Design review of the part built by this model. Coordinates are the model's own, in mm. A direction names the side the tool comes from. Round coordinates to 2 decimals unless told otherwise and drop trailing zeros. Write each loop counter-clockwise with the first axis right and the second up, starting at its lowest first coordinate (ties: lowest second). Pieces come first, ordered by that corner, then holes. Notation, with made-up numbers: (78.25, 71.5) -> (83.25, 71.5) arc R18 ccw to (83.25, 99.5) -> close; hole circle Ø8 at (74, 39). An arc over 180 degrees is marked (long way). One line per question, with ' | ' between items. Start each with the question number.
1) For faces 1 (the flat face through (103, 101.6, 25)), 2 (the conical face through (17.542, 17.713, 1.708)), list the 3-axis set-ups (+Z, -Z, +X, -X, +Y, -Y) from which the entire face can be reached by the end or side of a thin tool; tool diameter is ignored.
2) Consider section B-B (x = 86.5). Give the boundary of the cut face in (y, z) (3 decimals), then the cut area to 3 significant figures.
3) For probe 1 along Z at (x, y) = (105, 25.5); probe 2 along Z at (x, y) = (78, 87.5); probe 3 along Y at (x, z) = (35, 48.5), list the stretches that pass through material, from the lowest coordinate up.
4) Insertion check: pin 1 Ø1 at (x, y) = (156, 29) entering from -Z. The pin has a flat end and moves straight along its axis. Give the tip position at first contact, or say it passes through.
5) Consider section A-A (y = 58). Give the boundary of the cut face in (x, z) (3 decimals).
6) Mouldability with a two-part tool opening along X and no side actions: class faces 3 (the flat face through (0, 51, 25)), 4 (the flat face through (100, 51, 2.032)), 5 (the flat face through (100, 51, 50.8)) as +X half, -X half, draft (parallel to the pull), parting line (faces both ways), or undercut.
```python
from build123d import *

# Parameters (mm, degrees)
F1_DEPTH = 50.8
F2_R     = 3.175
F3_R     = 3.175
F4_DEPTH = 2.032
F4_TAPER = 45


with BuildPart() as f1:
    # F0 (on Top) → F1 (new body)
    with BuildSketch(Plane.XY):
        with BuildLine():
            ThreePointArc((0, 3.175), (0.9299359697, 0.9299359697), (3.175, 0))
            Line((3.175, 0), (200.025, 0))
            ThreePointArc((200.025, 0), (202.2700640303, 0.9299359697), (203.2, 3.175))
            Line((203.2, 3.175), (203.2, 98.425))
            ThreePointArc((203.2, 98.425), (202.2700640303, 100.6700640303), (200.025, 101.6))
            Line((200.025, 101.6), (3.175, 101.6))
            ThreePointArc((3.175, 101.6), (0.9299359697, 100.6700640303), (0, 98.425))
            Line((0, 98.425), (0, 3.175))
        make_face()
        with BuildLine():
            ThreePointArc((12.7000001431, 76.1999998569), (16.419744022, 85.180255978), (25.4000001431, 88.8999998569))
            Line((25.4000001431, 88.8999998569), (177.7999998569, 88.8999998569))
            ThreePointArc((177.7999998569, 88.8999998569), (186.780255978, 85.180255978), (190.4999998569, 76.1999998569))
            Line((190.4999998569, 76.1999998569), (190.4999998569, 25.4000001431))
            ThreePointArc((190.4999998569, 25.4000001431), (186.780255978, 16.419744022), (177.7999998569, 12.7000001431))
            Line((177.7999998569, 12.7000001431), (25.4000001431, 12.7000001431))
            ThreePointArc((25.4000001431, 12.7000001431), (16.419744022, 16.419744022), (12.7000001431, 25.4000001431))
            Line((12.7000001431, 25.4000001431), (12.7000001431, 76.1999998569))
        make_face(mode=Mode.SUBTRACT)
        with BuildLine():
            Line((177.7999998569, 88.8999998569), (25.4000001431, 88.8999998569))
            ThreePointArc((25.4000001431, 88.8999998569), (16.419744022, 85.180255978), (12.7000001431, 76.1999998569))
            Line((12.7000001431, 76.1999998569), (12.7000001431, 25.4000001431))
            ThreePointArc((12.7000001431, 25.4000001431), (16.419744022, 16.419744022), (25.4000001431, 12.7000001431))
            Line((25.4000001431, 12.7000001431), (177.7999998569, 12.7000001431))
            ThreePointArc((177.7999998569, 12.7000001431), (186.780255978, 16.419744022), (190.4999998569, 25.4000001431))
            Line((190.4999998569, 25.4000001431), (190.4999998569, 76.1999998569))
            ThreePointArc((190.4999998569, 76.1999998569), (186.780255978, 85.180255978), (177.7999998569, 88.8999998569))
        make_face()
    extrude(amount=F1_DEPTH)

    # F2
    f2_edges = [f1.edges().sort_by_distance(p)[0] for p in [
        (0, 50.8, 0),
        (0.929936, 0.929936, 0),
        (101.6, 0, 0),
        (202.270064, 0.929936, 0),
        (203.2, 50.8, 0),
        (202.270064, 100.670064, 0),
        (101.6, 101.6, 0),
        (0.929936, 100.670064, 0),
    ]]
    fillet(f2_edges, radius=F2_R)

    # F3
    f3_edges = [f1.edges().sort_by_distance(p)[0] for p in [
        (0, 50.8, 50.8),
        (0.929936, 0.929936, 50.8),
        (101.6, 0, 50.8),
        (202.270064, 0.929936, 50.8),
        (203.2, 50.8, 50.8),
        (202.270064, 100.670064, 50.8),
        (101.6, 101.6, 50.8),
        (0.929936, 100.670064, 50.8),
    ]]
    fillet(f3_edges, radius=F3_R)

    # F0 (on Top) → F4 (cut)
    with BuildSketch(Plane.XY):
        with BuildLine():
            Line((177.7999998569, 88.8999998569), (25.4000001431, 88.8999998569))
            ThreePointArc((25.4000001431, 88.8999998569), (16.419744022, 85.180255978), (12.7000001431, 76.1999998569))
            Line((12.7000001431, 76.1999998569), (12.7000001431, 25.4000001431))
            ThreePointArc((12.7000001431, 25.4000001431), (16.419744022, 16.419744022), (25.4000001431, 12.7000001431))
            Line((25.4000001431, 12.7000001431), (177.7999998569, 12.7000001431))
            ThreePointArc((177.7999998569, 12.7000001431), (186.780255978, 16.419744022), (190.4999998569, 25.4000001431))
            Line((190.4999998569, 25.4000001431), (190.4999998569, 76.1999998569))
            ThreePointArc((190.4999998569, 76.1999998569), (186.780255978, 85.180255978), (177.7999998569, 88.8999998569))
        make_face()
    extrude(amount=F4_DEPTH, taper=F4_TAPER, mode=Mode.SUBTRACT)


solid = f1.part
```
From the geometry:
1) face 1: +Z, -Z, +X, -X, +Y | face 2: -Z
2) outline: (0, 3.175) arc R3.175 ccw to (3.175, 0) -> (12.7, 0) -> (14.732, 2.032) -> (86.868, 2.032) -> (88.9, 0) -> (98.425, 0) arc R3.175 ccw to (101.6, 3.175) -> (101.6, 47.625) arc R3.175 ccw to (98.425, 50.8) -> (3.175, 50.8) arc R3.175 ccw to (0, 47.625) -> close | area: 5,000 mm2
3) probe 1: z = 2.03 to 50.8 | probe 2: z = 1.4 to 50.8 | probe 3: y = 0.12 to 101.48
4) pin 1: stops at z = 2.03
5) outline: (0, 3.175) arc R3.175 ccw to (3.175, 0) -> (12.7, 0) -> (14.732, 2.032) -> (188.468, 2.032) -> (190.5, 0) -> (200.025, 0) arc R3.175 ccw to (203.2, 3.175) -> (203.2, 47.625) arc R3.175 ccw to (200.025, 50.8) -> (3.175, 50.8) arc R3.175 ccw to (0, 47.625) -> close
6) face 3: -X half | face 4: undercut | face 5: draft
